Build history of the part. All positions in model axes, mm. Face numbers are marked on the shaded views. A direction names the side the tool comes from. Round coordinates to 2 decimals unless told otherwise and drop trailing zeros. Order: outer loops, then holes, each group sorted by start corner. A loop starts at its lowest first (then second) coordinate and runs counter-clockwise, first axis right, second up. Notation, with made-up numbers: (83, 16.25) -> (97, 16.25) arc R34 ccw to (97, 49.25) -> close; hole circle Ø5 at (28, -3.5). An arc over 180 degrees is marked (long way). Answer as a JSON object with one key per item and string values.
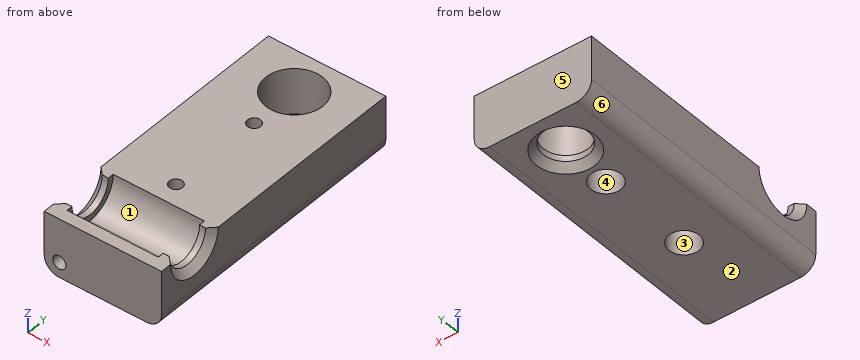
from build123d import *

# Parameters (mm, degrees)
F0_W      = 30.8750208
F0_H      = 72.8625058
F0_R      = 1.7272
F0_R_2    = 5.9124977
F1_DEPTH  = 3.437509
F2_W      = 30.8750208
F2_H      = 72.8625058
F2_R      = 1.7272
F2_R_2    = 7.5
F3_DEPTH  = 12
F4_W      = 24
F4_H      = 15
F5_DEPTH  = 7.5
F6_R      = 7.49999
F8_DEPTH  = 30.8750208
F9_R      = 3.96875
F10_DEPTH = 9.0875104
F11_R     = 3.96875
F12_R     = 1.7272
F13_DEPTH = 6.35
F14_SIZE  = 1.850009


# Not quite as in the source:
# - a fillet or chamfer is up to 0.001 mm smaller than in the source, because OpenCascade refuses the exact size


with BuildPart() as f1:
    # F0 (on Top) → F1 (new body)
    with BuildSketch(Plane.XY):
        with Locations((15.4375104, -36.4312529)):
            Rectangle(F0_W, F0_H)
        with Locations((15.4375104, -49.1312477)):
            Circle(F0_R, mode=Mode.SUBTRACT)
        with Locations((15.4375104, -23.7312477)):
            Circle(F0_R, mode=Mode.SUBTRACT)
        with Locations((15.4375104, -10.6749977)):
            Circle(F0_R_2, mode=Mode.SUBTRACT)
    extrude(amount=F1_DEPTH)

    # F2 (on face) → F3 (join)
    with BuildSketch(Plane.XY.offset(3.437509)):
        with Locations((15.4375104, -36.4312529)):
            Rectangle(F2_W, F2_H)
        with Locations((15.4375104, -49.1312477)):
            Circle(F2_R, mode=Mode.SUBTRACT)
        with Locations((15.4375104, -23.7312477)):
            Circle(F2_R, mode=Mode.SUBTRACT)
        with Locations((15.4375104, -10.6749977)):
            Circle(F2_R_2, mode=Mode.SUBTRACT)
    extrude(amount=F3_DEPTH)

    # F4 (on face) → F5 (cut)
    with BuildSketch(Plane.XY.offset(15.437509)):
        with Locations((15.4375104, -62.1875058)):
            Rectangle(F4_W, F4_H)
    extrude(amount=-F5_DEPTH, mode=Mode.SUBTRACT)

    # F6 (radius 7.5 in the source; OpenCascade refuses exactly that, so slightly less here)
    f6_edges = [f1.edges().sort_by_distance(p)[0] for p in [
        (15.43751, -54.687506, 7.937509),
        (15.43751, -69.687506, 7.937509),
    ]]
    fillet(f6_edges, radius=F6_R)

    # F7 (on face) → F8 (cut, through all)
    with BuildSketch(Plane(origin=(0, 0, 0), x_dir=(0, -1, 0), z_dir=(-1, 0, 0))):
        with BuildLine():
            Line((68.1000035, 15.437509), (56.2750081, 15.437509))
            ThreePointArc((56.2750081, 15.437509), (62.1875058, 9.5250113), (68.1000035, 15.437509))
        make_face()
    extrude(amount=-F8_DEPTH, mode=Mode.SUBTRACT)

    # F9 (on face) → F10 (cut)
    with BuildSketch(Plane(origin=(0, 0, 0), x_dir=(1, 0, 0), z_dir=(0, 0, -1))):
        with Locations((15.4375104, 23.7312477)):
            Circle(F9_R)
        with Locations((15.4375104, 49.1312477)):
            Circle(F9_R)
    extrude(amount=-F10_DEPTH, mode=Mode.SUBTRACT)

    # F11
    f11_edges = [f1.edges().sort_by_distance(p)[0] for p in [
        (0, -36.431253, 0),
        (30.875021, -36.431253, 0),
    ]]
    fillet(f11_edges, radius=F11_R)

    # F12 (on face) → F13 (cut)
    with BuildSketch(Plane.XZ.offset(72.8625058)):
        with Locations((3.96875, 3.96875)):
            Circle(F12_R)
    extrude(amount=-F13_DEPTH, mode=Mode.SUBTRACT)

    # F14
    f14_edges = [f1.edges().sort_by_distance(p)[0] for p in [
        (9.525013, -10.674998, 0),
        (30.875021, -62.187506, 9.525011),
        (0, -62.187506, 9.525011),
    ]]
    chamfer(f14_edges, length=F14_SIZE)


solid = f1.part
1) Pull direction X, two halves, no side cores. Call the marked faces 4, 5 and 6: pulls with the +X half, pulls with the -X half, needs draft (parallel to the pull), parting line crosses it, or undercut.
Checked values:
{"face 4": "undercut", "face 5": "needs draft", "face 6": "pulls with the -X half"}
2) Which spindle directions (+Z, -Z, +X, -X, +Y, -Y) get a long thin tool onto all of the face, cutting with end or side? Do the marked faces 1, 2 and 3. Say none if no direction does.
Checked values:
{"face 1": "+Z", "face 2": "-Z, +X, -X, +Y, -Y", "face 3": "-Z"}
3) Cut at D-D, the plane y = -27. Give the cut face in (x, z), plus the area to 3 significant figures.
Checked values:
{"outline": "(0, 3.97) arc R3.97 ccw to (3.97, 0) -> (13.19, 0) -> (13.19, 9.09) -> (17.69, 9.09) -> (17.69, 0) -> (26.91, 0) arc R3.97 ccw to (30.88, 3.97) -> (30.88, 15.44) -> (0, 15.44) -> close", "area": "429 mm²"}
4) Probe L1, parallel to Y at x = 14, z = 7; L2, parallel to Y at x = 12, z = 2.5; L3, parallel to Y at x = 5.5, z = 12. List the from-to ranges inside material, lowest first. Write a range as from..to.
Checked values:
{"L1": "y = -72.86..-52.83, -45.43..-27.43, -20.03..-18.04, -3.31..0", "L2": "y = -72.86..-51.11, -47.15..-25.71, -21.75..-15.49, -5.86..0", "L3": "y = -72.86..-68.85, -55.52..0"}
5) Cut at B-B, the plane z = 1. Give the cut face in (x, y) (1 decimal), plus the area to 3 significant figures.
Checked values:
{"outline": "(1.3, -72.9) -> (29.5, -72.9) -> (29.5, 0) -> (1.3, 0) -> close; hole circle Ø13.5 at (15.4, -10.7); hole circle Ø7.9 at (15.4, -49.1); hole circle Ø7.9 at (15.4, -23.7)", "area": "1,810 mm²"}
6) Flat gauge pins, fed straight in: pin 1 Ø9 at (x, y) = (15.44, -10.67) entering from -Z; pin 2 Ø5 at (x, y) = (15.44, -49.13) entering from -Z; pin 3 Ø4 at (y, z) = (-64.5, 12) entering from +X; pin 4 Ø4 at (y, z) = (-63, 10) entering from -X. Where does each tip first touch, or does it go through?
Checked values:
{"pin 1": "passes through", "pin 2": "stops at z = 9.09", "pin 3": "stops at x = 29.26", "pin 4": "stops at x = 0.26"}
7) Cut at C-C, the plane z = 14. Count the separate pieces of the cut face and the enclosed holes in it, plus the area to 3 significant figures.
Checked values:
{"separate pieces": "2", "enclosed holes": "3", "area": "1,610 mm²"}
